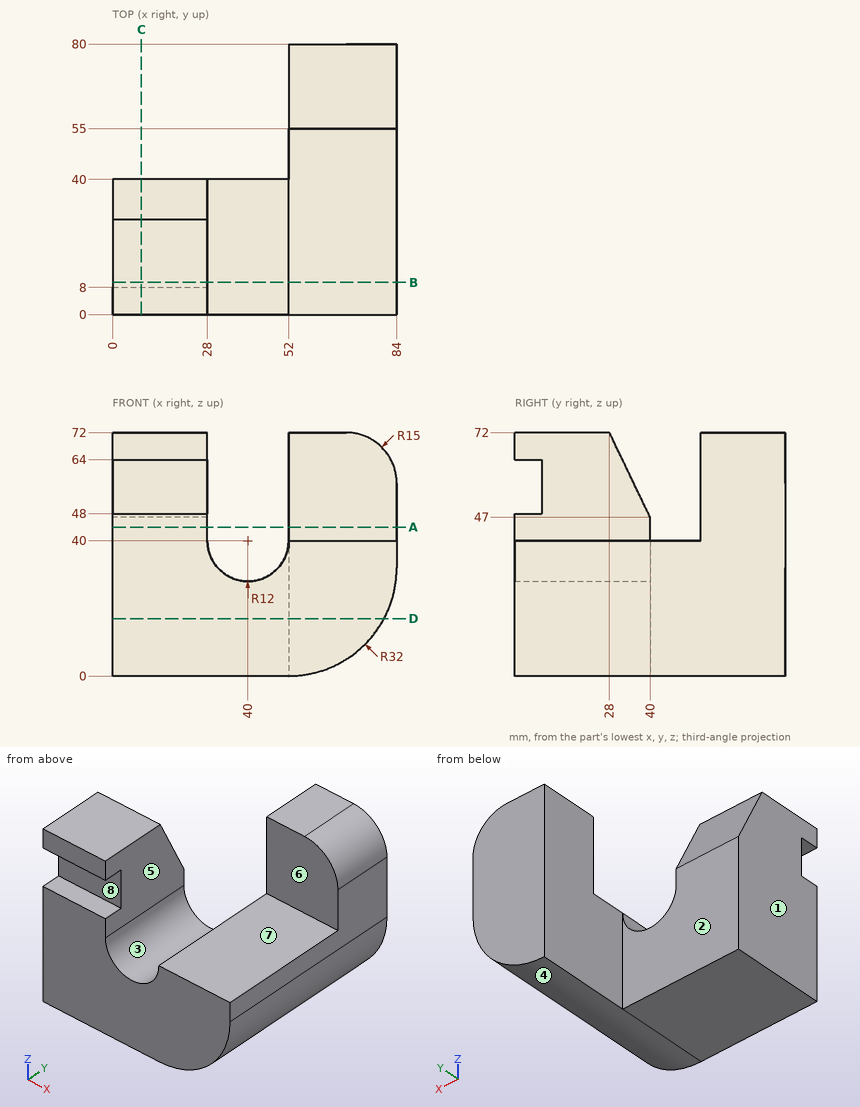
Check sheet for the drawn part. Datum: minimum x, y, z corner. Units: mm. A direction names the side the tool comes from. Coordinates: 2 decimals unless noted, no trailing zeros. Loops run counter-clockwise (first coordinate to the right, second up) from the corner with the lowest first, then second, coordinate; pieces in that order, holes last. Notation, with made-up numbers: (-39.5, 7.25) -> (-16.5, 7.25) arc R23 cw to (-16.5, 18.25) -> close; hole circle Ø5 at (17, -35.75). An arc over 180 degrees is marked (long way). Answer in a Markdown table with one row per item.
1. Sectioned sample at D-D, the plane z = 17. Record the boundary of the cut face in (x, y).
Check values:
| item | result |
|---|---|
| outline | (0, 0) -> (80.27, 0) -> (80.27, 80) -> (52, 80) -> (52, 40) -> (0, 40) -> close |
2. Go/stop test with flat-tipped pins: pin 1 (2 mm diameter, centred on y = 50.5, z = 11.5, fed in from +X); pin 2 (3 mm diameter, centred on x = 66.5, y = 24.5, fed in from +Z); pin 3 (23.5 mm diameter, centred on x = 33.5, z = 28.5, fed in from +Y). Record where each tip stops, or that it passes through.
Check values:
| item | result |
|---|---|
| pin 1 | stops at x = 77.37 |
| pin 2 | stops at z = 40 |
| pin 3 | stops at y = 40 |
3. Sectioned sample at B-B, the plane y = 9.5. Record the boundary of the cut face in (x, z), then the cut area to 3 significant figures.
Check values:
| item | result |
|---|---|
| outline | (0, 0) -> (52, 0) arc R32 ccw to (84, 32) -> (84, 40) -> (52, 40) arc R12 cw to (28, 40) -> (28, 72) -> (0, 72) -> close |
| area | 3,810 mm2 |
4. Access from +Z, -Z, +X, -X, +Y, -Y to the whole of each face (thin tool, end or side, straight path). Record for the marked faces 5, 6, 7 and 8.
Check values:
| item | result |
|---|---|
| face 5 | +Z, +X, +Y, -Y |
| face 6 | +Z, +X, -X, -Y |
| face 7 | +Z, +X, -Y |
| face 8 | +X, -X, -Y |
5. Sectioned sample at C-C, the plane x = 8.5. Record the boundary of the cut face in (y, z), then the cut area to 3 significant figures.
Check values:
| item | result |
|---|---|
| outline | (0, 0) -> (40, 0) -> (40, 47) -> (28, 72) -> (0, 72) -> (0, 64) -> (8, 64) -> (8, 48) -> (0, 48) -> close |
| area | 2,600 mm2 |
6. Sectioned sample at A-A, the plane z = 44. Record the boundary of the cut face in (x, y).
Check values:
| item | result |
|---|---|
| outline | (0, 0) -> (28, 0) -> (28, 40) -> (0, 40) -> close; (52, 55) -> (84, 55) -> (84, 80) -> (52, 80) -> close |
7. Material ranges on line 1 along Z through (x, y) = (20, 6.5); line 2 along X through (y, z) = (17, 54); line 3 along X through (y, z) = (38, 29), recorded low to high. Write a range as [from, to].
Check values:
| item | result |
|---|---|
| line 1 | z = [0, 48], [64, 72] |
| line 2 | x = [0, 28] |
| line 3 | x = [0, 35.2], [44.8, 83.86] |
8. Release check for a two-part mould opening along X. For the marked faces 1, 2, 3 and 4 record: released by +X, released by -X, zero draft, split by the parting line, or undercut.
Check values:
| item | result |
|---|---|
| face 1 | released by -X |
| face 2 | zero draft |
| face 3 | undercut |
| face 4 | released by +X |
